from build123d import *

# Parameters (mm, degrees)
SKETCH_1_R                  = 26
EXTRUDE_1_DEPTH             = 14
CUT_EXTRUDE_1_DEPTH         = 30
SKETCH_4_R                  = 4.5
CUT_EXTRUDE_2_DEPTH         = 40.344631146
CUT_EXTRUDE_3_DEPTH         = 12
HOLE_WIZARD_M31_D           = 3.4
HOLE_WIZARD_M31_CBORE_D     = 6
HOLE_WIZARD_M31_CBORE_DEPTH = 3.2
EXTRUDE_START               = 15
SKETCH_12_R                 = 26
SKETCH_12_R_2               = 24
EXTRUDE_2_DEPTH             = 15


with BuildPart() as part:
    # Эскиз1 → Бобышка-Вытянуть1 (new body)
    with BuildSketch(Plane(origin=(0, 0, 0), x_dir=(1, 0, 0), z_dir=(0, 1, 0))):
        with Locations(Location((0, 0, 0), (0, 0, 270))):
            Circle(SKETCH_1_R)
    extrude(amount=EXTRUDE_1_DEPTH)

    # Эскиз2 → Вырез-Вытянуть1 (cut, symmetric)
    with BuildSketch(Plane(origin=(0, 0, 0), x_dir=(0, 0, -1), z_dir=(1, 0, 0))):
        Polygon((13.654700538, 6), (-13.654700538, 6), (-9.728718708, 12.8), (-9.728718708, 14), (9.728718708, 14), (9.728718708, 12.8), align=None)
    extrude(amount=CUT_EXTRUDE_1_DEPTH, both=True, mode=Mode.SUBTRACT)

    # Эскиз4 → Вырез-Вытянуть2 (cut, through all)
    with BuildSketch(Plane.XZ):
        with Locations(Location((0, 0, 0), (0, 0, 270))):
            Circle(SKETCH_4_R)
    extrude(amount=-CUT_EXTRUDE_2_DEPTH, mode=Mode.SUBTRACT)

    # Эскиз5 → Вырез-Вытянуть3 (cut)
    with BuildSketch(Plane.XZ):
        with BuildLine():
            Line((-18.05935633, -15.654700538), (18.05935633, -15.654700538))
            ThreePointArc((18.05935633, -15.654700538), (0, -23.9), (-18.05935633, -15.654700538))
        make_face()
    extrude(amount=-CUT_EXTRUDE_3_DEPTH, mode=Mode.SUBTRACT)

    # Цековка для винта с внутренним шестигранником M31 (through all)
    with Locations(Plane(origin=(0, 6, 0), x_dir=(1, 0, 0), z_dir=(0, 1, 0))):
        with Locations((-6.717514421, 6.717514421), (6.717514421, 6.717514421), (6.717514421, -6.717514421), (-6.717514421, -6.717514421)):
            CounterBoreHole(HOLE_WIZARD_M31_D / 2, HOLE_WIZARD_M31_CBORE_D / 2, HOLE_WIZARD_M31_CBORE_DEPTH)

    # Эскиз12 → Бобышка-Вытянуть2 (add)
    with BuildSketch(Plane.XZ.offset(EXTRUDE_START)):
        with Locations(Location((0, 0, 0), (0, 0, 270))):
            Circle(SKETCH_12_R)
        with Locations(Location((0, 0, 0), (0, 0, 270))):
            Circle(SKETCH_12_R_2, mode=Mode.SUBTRACT)
    extrude(amount=-EXTRUDE_2_DEPTH)


solid = part.part
The listing builds one solid part. Answer for the finished solid, in the listing's coordinates (mm). A direction names the side the tool comes from. Give positions to 0.01 mm unless a question says otherwise; leave off trailing zeros. Order: outer loops, then holes, each group sorted by start corner. A loop starts at its lowest first (then second) coordinate and runs counter-clockwise, first axis right, second up. Notation, with made-up numbers: (-3, -17) - (5, -17) arc R18 cw to (5, 16) - close; hole circle Ø11 at (-13.75, 30.25). An arc over 180 degrees is marked (long way). One line per item, written item: value. Start each with the question number.
1) The mould has two halves that part along Z. Classify faces 5 (the face through (0, 13, -9.729)), 6 (the face through (0, 14, 16)): released by +Z, released by -Z, zero draft, split by the parting line, or undercut.
2) A cutting plane is placed at D-D on z = -7.5. Give the vertices of the cut face in (x, y).
3) A cutting plane is placed at C-C on y = 4.5. Give the vertices of the cut face in (x, z), then the cut area to 3 significant figures.
4) Given pin 1 Ø1.5 at (x, z) = (19.5, 7) entering from +Y; pin 2 Ø3 at (x, z) = (-8, -6) entering from +Y; pin 3 Ø1 at (y, z) = (-1, 6) entering from +X; pin 4 Ø2.5 at (x, z) = (6.72, -6.72) entering from -Y, each flat-ended and moving along its own axis, determine where each tip first touches the part or whether it passes through.
5) Find the intervals of material crossed by L1, parallel to X at y = -8.5, z = 0; L2, parallel to X at y = 4, z = -7; L3, parallel to Z at x = -2, y = 10.5, in increasing order.
6) A cutting plane is placed at B-B on x = 0. Give the vertices of the cut face in (y, z).
7) A tool of negligible diameter and unlimited length cuts with its end or side. For faces 1 (the face through (0, 13, 9.729)), 2 (the face through (-5, 6, 0)), 3 (the face through (-9.715, 4.422, -6.849)), 4 (the face through (0, 12, -19)), from which of +Z, -Z, +X, -X, +Y, -Y can it reach the whole face along a straight path? Write none if from no direction.
8) A cutting plane is placed at A-A on z = 0. Give the vertices of the cut face in (x, y).
Answer sheet:
1. face 5: undercut
1. face 6: zero draft
2. outline: (-24.89, -15) - (-22.8, -15) - (-22.8, 0) - (-8.23, 0) - (-8.23, 2.8) - (-9.61, 2.8) - (-9.61, 6) - (-24.89, 6) - close; (-5.21, 0) - (5.21, 0) - (5.21, 2.8) - (3.82, 2.8) - (3.82, 6) - (-3.82, 6) - (-3.82, 2.8) - (-5.21, 2.8) - close; (8.23, 0) - (22.8, 0) - (22.8, -15) - (24.89, -15) - (24.89, 6) - (9.61, 6) - (9.61, 2.8) - (8.23, 2.8) - close
3. outline: circle Ø52 at (0, 0); hole (-18.06, -15.65) arc R23.9 ccw to (18.06, -15.65) - close; hole circle Ø6 at (-6.72, -6.72); hole circle Ø6 at (-6.72, 6.72); hole circle Ø9 at (0, 0); hole circle Ø6 at (6.72, -6.72); hole circle Ø6 at (6.72, 6.72)
3. area: 1,740 mm2
4. pin 1: stops at y = 6
4. pin 2: stops at y = 2.8
4. pin 3: stops at x = 25.41
4. pin 4: passes through
5. L1: x = -26 to -24, 24 to 26
5. L2: x = -25.04 to -9.7, -3.73 to 3.73, 9.7 to 25.04
5. L3: z = -25.92 to -23.82, -15.65 to -11.06, 11.06 to 25.92
6. outline: (-15, -26) - (14, -26) - (14, -9.73) - (12.8, -9.73) - (6, -13.65) - (6, -4.5) - (0, -4.5) - (0, -15.65) - (12, -15.65) - (12, -23.9) - (0, -23.9) - (0, -24) - (-15, -24) - close; (-15, 24) - (0, 24) - (0, 4.5) - (6, 4.5) - (6, 13.65) - (12.8, 9.73) - (14, 9.73) - (14, 26) - (-15, 26) - close
7. face 1: +X, -X, +Y
7. face 2: +X, -X
7. face 3: +Y
7. face 4: -Y
8. outline: (-26, -15) - (-24, -15) - (-24, 0) - (-4.5, 0) - (-4.5, 6) - (-26, 6) - close; (4.5, 0) - (24, 0) - (24, -15) - (26, -15) - (26, 6) - (4.5, 6) - close
